Source: CAD feature listing. Evaluate the final solid. Frame: model axes, mm. A direction names the side the tool comes from. Round coordinates to 2 decimals unless told otherwise and drop trailing zeros. Loops run counter-clockwise (first coordinate to the right, second up) from the corner with the lowest first, then second, coordinate; pieces in that order, holes last. Notation, with made-up numbers: (26.25, 44) -> (31.25, 44) arc R12 ccw to (31.25, 66) -> close; hole circle Ø3 at (-7.5, -12.75). An arc over 180 degrees is marked (long way). Return JSON: item names as keys, results as strings. Group by question number.
```python
from build123d import *

# Parameters (mm, degrees)
SKETCH1_W           = 44.45
SKETCH1_H           = 6.35
BOSS_EXTRUDE1_DEPTH = 6.35


with BuildPart() as part:
    # Sketch1 → Boss-Extrude1 (new body)
    with BuildSketch(Plane.XY):
        Polygon((0, -98.986703653), (152.4, -98.986703653), (161.925, -82.48891971), (9.525, 181.475623363), (-9.525, 181.475623363), (-161.925, -82.48891971), (-152.4, -98.986703653), align=None)
        with BuildLine():
            Line((-3.302, 166.995927543), (3.302, 166.995927543))
            Line((3.302, 166.995927543), (3.302, 44.428223237))
            ThreePointArc((3.302, 44.428223237), (4.471070917, 41.186150797), (7.440202247, 39.436288042))
            ThreePointArc((7.440202247, 39.436288042), (34.755331505, 20.066), (37.872928399, -13.274739866))
            ThreePointArc((37.872928399, -13.274739866), (37.903788333, -16.721014402), (40.126969968, -19.354495735))
            Line((40.126969968, -19.354495735), (146.273715581, -80.638347888))
            Line((146.273715581, -80.638347888), (142.971715581, -86.357579655))
            Line((142.971715581, -86.357579655), (36.824969968, -25.073727502))
            ThreePointArc((36.824969968, -25.073727502), (33.432717416, -24.465136395), (30.432726152, -26.161548176))
            ThreePointArc((30.432726152, -26.161548176), (0, -40.132), (-30.432726152, -26.161548176))
            ThreePointArc((-30.432726152, -26.161548176), (-33.432717416, -24.465136395), (-36.824969968, -25.073727502))
            Line((-36.824969968, -25.073727502), (-142.971715581, -86.357579655))
            Line((-142.971715581, -86.357579655), (-146.273715581, -80.638347888))
            Line((-146.273715581, -80.638347888), (-40.126969968, -19.354495735))
            ThreePointArc((-40.126969968, -19.354495735), (-37.903788333, -16.721014402), (-37.872928399, -13.274739866))
            ThreePointArc((-37.872928399, -13.274739866), (-34.755331505, 20.066), (-7.440202247, 39.436288042))
            ThreePointArc((-7.440202247, 39.436288042), (-4.471070917, 41.186150797), (-3.302, 44.428223237))
            Line((-3.302, 44.428223237), (-3.302, 166.995927543))
        make_face(mode=Mode.SUBTRACT)
        with Locations((0, -79.936703653)):
            Rectangle(SKETCH1_W, SKETCH1_H, mode=Mode.SUBTRACT)
        Polygon((-83.089346715, 22.308437227), (-60.864346715, 60.803266425), (-55.365085401, 57.628266425), (-77.590085401, 19.133437227), align=None, mode=Mode.SUBTRACT)
        Polygon((60.864346715, 60.803266425), (55.365085401, 57.628266425), (77.590085401, 19.133437227), (83.089346715, 22.308437227), align=None, mode=Mode.SUBTRACT)
    extrude(amount=BOSS_EXTRUDE1_DEPTH)


solid = part.part
```
(1) Cut plane C-C (x = 121.5). Return loops of the section in (y, z).
(2) Set-up query: faces 1 (the face through (0.48, -40.13, 3.13)), 2 (the face through (-84.66, 51.34, 3.13)). Return all of +Z, -Z, +X, -X, +Y, -Y with unobstructed straight access to the full face (end or side cutting, diameter ignored); none if empty.
(3) Pin query (flat end, axial travel): pin 1 (1.5 mm diameter, centred on y = 146.5, z = 4, fed in from +X). Return the tip coordinate at first contact, or that it passes through.
(4) Ray query, line 1 (Y direction, x = 79, z = 4.25); line 2 (X direction, y = 53, z = 6.25); line 3 (X direction, y = 19.5, z = 4.75) (3 decimals). Return the intervals inside material, ascending.
(5) Cut plane B-B (y = 110.5). Return loops of the section in (x, z), and give its area (3 significant figures).
(6) Cut plane D-D (y = 33). Return loops of the section in (x, z).
(7) Cut plane A-A (x = 72). Return loops of the section in (y, z).
(8) Mould query, pull axis Y, two halves, no side actions, for faces 3 (the face through (92.46, -49.57, 3.13)), 4 (the face through (-2, -50, 6.35)), 5 (the face through (86.79, 47.65, 3.13)), 6 (the face through (-157.23, -90.62, 3.13)). Classes: released by +Y, released by -Y, zero draft, split by the parting line, or undercut.
Answers follow:
{
 "1": {"outline": "(-98.99, 0) -> (-73.96, 0) -> (-73.96, 6.35) -> (-98.99, 6.35) -> close; (-66.34, 0) -> (-12.47, 0) -> (-12.47, 6.35) -> (-66.34, 6.35) -> close"},
 "2": {"face 1": "+Z, -Z", "face 2": "+Z, -Z, -X, +Y"},
 "3": {"pin 1": "x = 30.15"},
 "4": {"line 1": "-98.99 to -49.42, -41.8 to 19.95, 29.39 to 61.14", "line 2": "-83.7 to -65.37, -58.04 to -3.3, 3.3 to 58.04, 65.37 to 83.7", "line 3": "-103.042 to -78.225, -77.378 to -35.076, 35.076 to 77.378, 78.225 to 103.042"},
 "5": {"outline": "(-50.5, 0) -> (-3.3, 0) -> (-3.3, 6.35) -> (-50.5, 6.35) -> close; (3.3, 0) -> (50.5, 0) -> (50.5, 6.35) -> (3.3, 6.35) -> close", "area": "599 mm^2"},
 "6": {"outline": "(-95.25, 0) -> (-76.92, 0) -> (-76.92, 6.35) -> (-95.25, 6.35) -> close; (-69.58, 0) -> (-22.84, 0) -> (-22.84, 6.35) -> (-69.58, 6.35) -> close; (22.84, 0) -> (69.58, 0) -> (69.58, 6.35) -> (22.84, 6.35) -> close; (76.92, 0) -> (95.25, 0) -> (95.25, 6.35) -> (76.92, 6.35) -> close"},
 "7": {"outline": "(-98.99, 0) -> (-45.38, 0) -> (-45.38, 6.35) -> (-98.99, 6.35) -> close; (-37.76, 0) -> (28.82, 0) -> (28.82, 6.35) -> (-37.76, 6.35) -> close; (41.52, 0) -> (73.27, 0) -> (73.27, 6.35) -> (41.52, 6.35) -> close"},
 "8": {"face 3": "undercut", "face 4": "zero draft", "face 5": "released by +Y", "face 6": "released by -Y"}
}
